Source: CAD feature listing. Evaluate the final solid. Frame: model axes, mm. A direction names the side the tool comes from. Round coordinates to 2 decimals unless told otherwise and drop trailing zeros. Order: outer loops, then holes, each group sorted by start corner. A loop starts at its lowest first (then second) coordinate and runs counter-clockwise, first axis right, second up. Notation, with made-up numbers: (78.25, 62.5) - (94.25, 62.5) arc R31 cw to (94.25, 97.5) - close; hole circle Ø1 at (-5.75, -13.5). An arc over 180 degrees is marked (long way). Put each result on its own line as item: value. Start each with the question number.
1) Section A-A on z = 5.75. Output: boundary loops of the cut face in (x, y) (3 decimals), then the cut area to 3 significant figures.
2) Contact query for flat-ended pins moving along their axis: P1, Ø8, axis at x = 16.5, y = 4.5, coming from the +Z side; P2, Ø2.5, axis at x = 13, z = 4.5, coming from the -Y side; P3, Ø4, axis at y = 5, z = 6, coming from the +X side; P4, Ø6, axis at x = 14, y = 2, coming from the +Z side. Output: stop coordinate, or through.
3) Section B-B on y = 6. Output: boundary loops of the cut face in (x, z), then the cut area to 3 significant figures.
4) Line query: probe 1 along X at (y, z) = (6.5, 2.25); probe 2 along Y at (x, z) = (15.75, 3.25); probe 3 along X at (y, z) = (9, 3.5). Output: solid intervals per line, ascending. Write a range as [from, to].
5) Access query for faces 1 (the face through (14, 5.334, 5)), 2 (the face through (14, 8, 2.921)), 3 (the face through (14, 8, 6.096)). Directions: +Z, -Z, +X, -X, +Y, -Y. A direction counts if a zero-diameter tool reaches every point of the face in a straight line with its end or side. Return the directions, or none.
6) Section C-C on x = 15.5. Output: boundary loops of the cut face in (y, z).
7) Section D-D on y = 13.25. Output: boundary loops of the cut face in (x, z), then the cut area to 3 significant figures.
Autodesk Inventor part; units mm, degrees
ref_plane "YZ Plane" through (0, 0, 0) normal (1, 0, 0) x (0, 1, 0)
ref_plane "XZ Plane" through (0, 0, 0) normal (0, 1, 0) x (-1, 0, 0)
ref_plane "XY Plane" through (0, 0, 0) normal (0, 0, 1) x (1, 0, 0)
sketch "Sketch1" plane through (0, 0, 0) normal (0, 0, 1) x (1, 0, 0)
  line L0 (0, 0) -> (10.16, 0)
  line L1 (10.16, 0) -> (10.16, 19.304)
  line L2 (10.16, 19.304) -> (0, 19.304)
  line L3 (0, 19.304) -> (0, 0)
  dimension "d0" = 10.16
  dimension "d1" = 19.304
extrude "Extrusion1" add sketch "Sketch1" along normal blind 7.9248
sketch "Sketch2" plane through (10.16, 0, 0) normal (1, 0, 0) x (0, 0, -1)
  line L0 (0, 0) -> (-7.9248, 0)
  line L1 (0, 0) -> (0, 19.304)
  line L2 (0, 19.304) -> (-7.9248, 19.304)
  line L3 (-2.921, 10.414) -> (-6.096, 10.414)
  line L4 (-6.096, 10.414) -> (-6.096, 5.334)
  line L5 (-6.096, 5.334) -> (-2.921, 5.334)
  line L6 (-2.921, 5.334) -> (-2.921, 10.414)
  line L7 (-6.096, 10.414) -> (-6.096, 13.97)
  line L8 (-6.096, 13.97) -> (-2.921, 13.97)
  line L9 (-2.921, 13.97) -> (-2.921, 10.414)
  dimension "d5" = 5.08
  dimension "d6" = 3.175
  dimension "d9" = 2.921
  dimension "d10" = 3.556
  dimension "d11" = 5.334
  dimension "d13" = 5.334
extrude "Extrusion2" add sketch "Sketch2" along normal blind 8.509 contours L6 L5 L4 L3
sketch "Sketch3" plane through (10.16, 5.334, 6.096) normal (0, 0, 1) x (1, 0, 0)
  line L0 (8.509, 0) -> (8.509, 5.08)
  line L1 (0, 5.08) -> (8.509, 5.08)
  line L2 (0, 0) -> (0, 5.08)
  line L3 (0, 0) -> (8.509, 0)
  arc A0 (7.7118, 0) -> (7.7118, 5.08) centre (4.064, 2.54) ccw
  point P0 (-10.16, -5.334)
  dimension "d17" = 4.445
extrude "Extrusion3" cut sketch "Sketch3" against normal through all contours L3 A0 L0 | A0 L1 L0
equation "\"d11\" = d13"
properties part number "power_switch"
Answer sheet:
1. outline: (0, 0) - (10.16, 0) - (10.16, 5.334) - (17.872, 5.334) arc R4.445 ccw to (17.872, 10.414) - (10.16, 10.414) - (10.16, 19.304) - (0, 19.304) - close
1. area: 238 mm^2
2. P1: z = 6.1
2. P2: y = 5.33
2. P3: x = 18.58
2. P4: through
3. outline: (0, 0) - (10.16, 0) - (10.16, 2.92) - (18.25, 2.92) - (18.25, 6.1) - (10.16, 6.1) - (10.16, 7.92) - (0, 7.92) - close
3. area: 106 mm^2
4. probe 1: [0, 10.16]
4. probe 2: [5.33, 10.41]
4. probe 3: [0, 18.52]
5. face 1: +Z, -Z, +X, -Y
5. face 2: -Z, +X, +Y, -Y
5. face 3: +Z, +X, +Y, -Y
6. outline: (5.33, 2.92) - (10.41, 2.92) - (10.41, 6.1) - (5.33, 6.1) - close
7. outline: (0, 0) - (10.16, 0) - (10.16, 7.92) - (0, 7.92) - close
7. area: 80.5 mm^2
